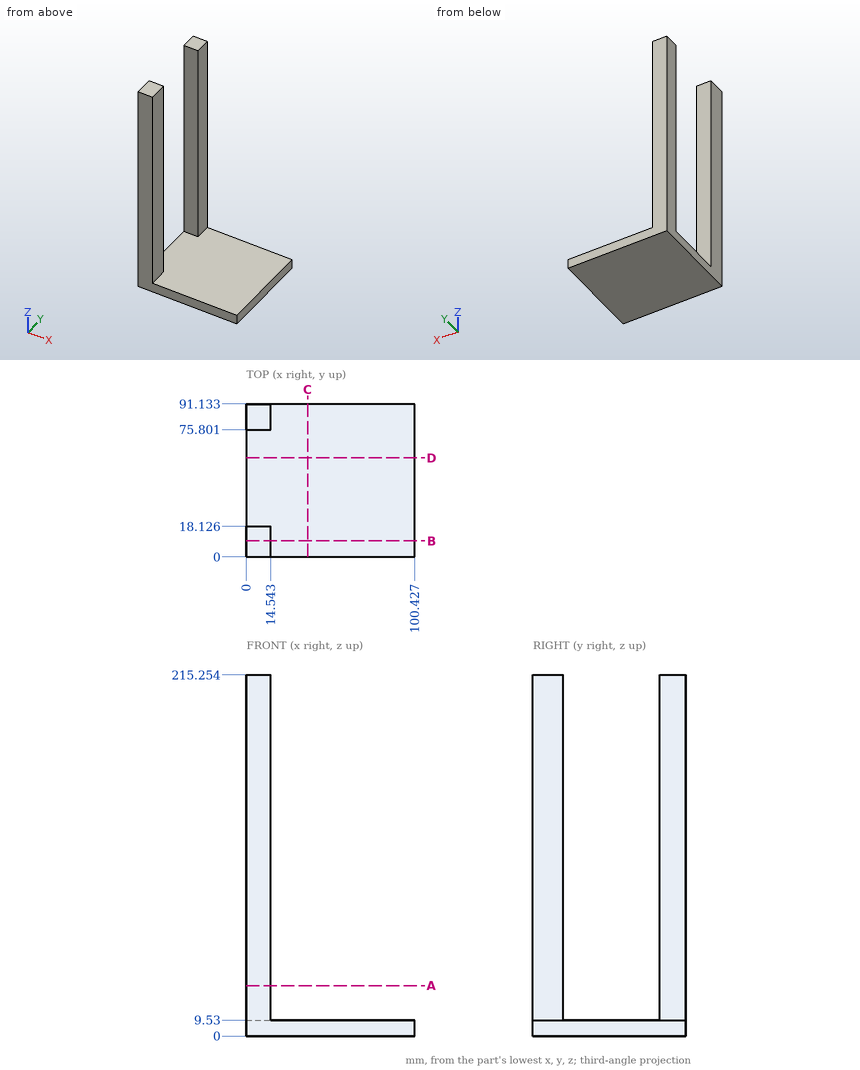
Could you check a few things on this drawing? It's one solid part, dimensions in mm from its lowest x, y, z. Round coordinates to 2 decimals unless told otherwise and drop trailing zeros. Order: outer loops, then holes, each group sorted by start corner. A loop starts at its lowest first (then second) coordinate and runs counter-clockwise, first axis right, second up. Notation, with made-up numbers: (87.25, -38.5) -> (133.25, -38.5) arc R27 cw to (133.25, -3.5) -> close; hole circle Ø11 at (68.5, -31). An arc over 180 degrees is marked (long way). One line per question, with ' | ' between items.
Q1. I'm going to push flat-ended pins straight in: pin 1 (12.5 mm diameter, centred on y = 83.5, z = 107, fed in from +X); pin 2 (1 mm diameter, centred on x = 41, y = 45.5, fed in from +Z). Where does each tip first touch, or does it pass through?
Computed values:
pin 1: x = 14.54 | pin 2: z = 9.53
Q2. If we section it at C-C on x = 36.5: Write out the boundary of the cut face in (y, z).
Computed values:
outline: (0, 0) -> (91.13, 0) -> (91.13, 9.53) -> (0, 9.53) -> close
Q3. If we section it at B-B on y = 9.5: Write out the boundary of the cut face in (x, z).
Computed values:
outline: (0, 0) -> (100.43, 0) -> (100.43, 9.53) -> (14.54, 9.53) -> (14.54, 215.25) -> (0, 215.25) -> close
Q4. If we section it at A-A on z = 30: Write out the boundary of the cut face in (x, y).
Computed values:
outline: (0, 0) -> (14.54, 0) -> (14.54, 18.13) -> (0, 18.13) -> close; (0, 75.8) -> (14.54, 75.8) -> (14.54, 91.13) -> (0, 91.13) -> close
Q5. If we section it at D-D on y = 59: Write out the boundary of the cut face in (x, z).
Computed values:
outline: (0, 0) -> (100.43, 0) -> (100.43, 9.53) -> (0, 9.53) -> close
Q6. If I drill on line 1 (Y direction, x = 6, z = 205); line 2 (Z direction, x = 41.5, y = 31.5); line 3 (X direction, y = 79, z = 121.5), over which ranges is the centre line in solid material (lowest first)? Write a range as from..to.
Computed values:
line 1: 0..18.13, 75.8..91.13 | line 2: 0..9.53 | line 3: 0..14.54
